Input: dimensioned drawing with shaded views. Units: mm. Origin: part minimum x, y, z. Coordinates: 2 decimals unless noted, no trailing zeros. Order: outer loops, then holes, each group sorted by start corner. A loop starts at its lowest first (then second) coordinate and runs counter-clockwise, first axis right, second up. Notation, with made-up numbers: (0, 20.25) - (44, 20.25) arc R19 cw to (44, 55.25) - close; hole circle Ø11 at (40, -25). An arc over 180 degrees is marked (long way). Answer as CSV lines item,"result". Start each with the question number.
Item 1: Section A-A (x = 28). Output: boundary loops of the cut face in (y, z).
Item 2: Material intervals for line 1 along Y through (x, z) = (34.5, 1.2); line 2 along Y through (x, z) = (23, 2.45); line 3 along X through (y, z) = (50, 2.1), sorted ascending.
Item 3: Section B-B (y = 53.5). Output: boundary loops of the cut face in (x, z).
Item 4: Section C-C (x = 1.5). Output: boundary loops of the cut face in (y, z), and give its area (3 significant figures).
Item 5: Section D-D (z = 0.85). Output: boundary loops of the cut face in (x, y).
Item 6: First-contact query: pin 1 (6 mm diameter, centred on x = 5, y = 59, fed in from +Z). Flat tip, straight axial feed; report the tip coordinate or a pass-through.
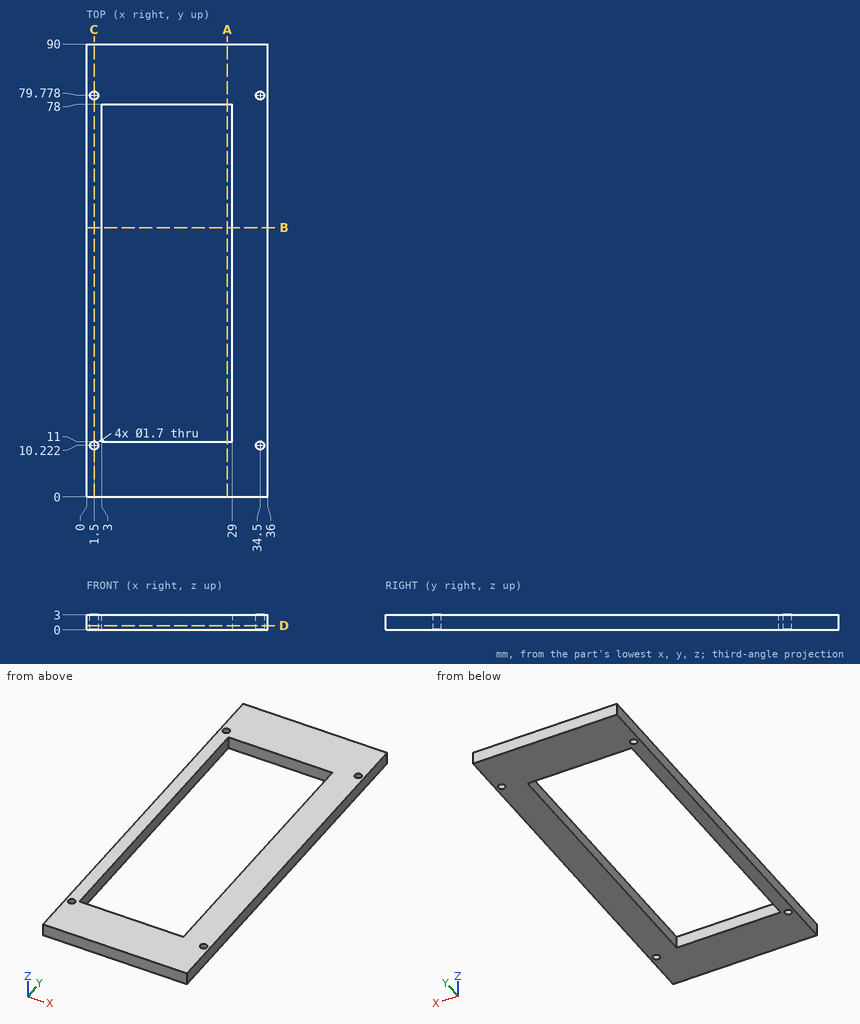
Determined:
1,outline,"(0, 0) - (11, 0) - (11, 3) - (0, 3) - close; (78, 0) - (90, 0) - (90, 3) - (78, 3) - close"
2,line 1,"y = 0 to 9.37, 11.07 to 78.93, 80.63 to 90"
2,line 2,"y = 0 to 11, 78 to 90"
2,line 3,"x = 0 to 3, 29 to 36"
3,outline,"(0, 0) - (3, 0) - (3, 3) - (0, 3) - close; (29, 0) - (36, 0) - (36, 3) - (29, 3) - close"
4,outline,"(0, 0) - (9.37, 0) - (9.37, 3) - (0, 3) - close; (11.07, 0) - (78.93, 0) - (78.93, 3) - (11.07, 3) - close; (80.63, 0) - (90, 0) - (90, 3) - (80.63, 3) - close"
4,area,"260 mm^2"
5,outline,"(0, 0) - (36, 0) - (36, 90) - (0, 90) - close; hole circle Ø1.7 at (1.5, 10.22); hole circle Ø1.7 at (1.5, 79.78); hole (3, 11) - (29, 11) - (29, 78) - (3, 78) - close; hole circle Ø1.7 at (34.5, 10.22); hole circle Ø1.7 at (34.5, 79.78)"
6,pin 1,"stops at z = 3"
